```python
from build123d import *

# Parameters (mm, degrees)
SKETCH_1_W          = 25
SKETCH_1_H          = 90
EXTRUDE_1_DEPTH     = 2
SKETCH_3_W          = 2
SKETCH_3_H          = 90
EXTRUDE_2_DEPTH     = 40
SKETCH_6_R          = 1.65
CUT_EXTRUDE_3_DEPTH = 10
SKETCH_7_R          = 3
CUT_EXTRUDE_4_DEPTH = 10
SKETCH_8_R          = 1.65
CUT_EXTRUDE_5_DEPTH = 10
EXTRUDE_3_DEPTH     = 27
SKETCH_10_R         = 1.65
SKETCH_10_R_2       = 2
CUT_EXTRUDE_7_DEPTH = 6


with BuildPart() as part:
    # 草图1 → 凸台-拉伸1 (new body)
    with BuildSketch(Plane(origin=(0, 0, 0), x_dir=(1, 0, 0), z_dir=(0, 1, 0))):
        Rectangle(SKETCH_1_W, SKETCH_1_H)
    extrude(amount=EXTRUDE_1_DEPTH)

    # 草图3 → 凸台-拉伸2 (add)
    with BuildSketch(Plane(origin=(0, 2, 0), x_dir=(1, 0, 0), z_dir=(0, 1, 0))):
        with Locations((-11.5, 0)):
            Rectangle(SKETCH_3_W, SKETCH_3_H)
    extrude(amount=EXTRUDE_2_DEPTH)

    # 草图6 → 切除-拉伸3 (cut)
    with BuildSketch(Plane.ZY.offset(12.5)):
        with Locations((8, 21)):
            Circle(SKETCH_6_R)
        with Locations((21.524795588, 17.383384964)):
            Circle(SKETCH_6_R)
        with Locations((15, 14)):
            Circle(SKETCH_6_R)
        with Locations((15, 28)):
            Circle(SKETCH_6_R)
    extrude(amount=-CUT_EXTRUDE_3_DEPTH, mode=Mode.SUBTRACT)

    # 草图7 → 切除-拉伸4 (cut)
    with BuildSketch(Plane(origin=(0, 0, 0), x_dir=(-1, 0, 0), z_dir=(0, -1, 0))):
        with Locations(Location((-4.5, 28.45, 0), (0, 0, 90))):
            Circle(SKETCH_7_R)
    extrude(amount=-CUT_EXTRUDE_4_DEPTH, mode=Mode.SUBTRACT)

    # 草图8 → 切除-拉伸5 (cut)
    with BuildSketch(Plane(origin=(-10.5, 0, 0), x_dir=(0, 0, -1), z_dir=(1, 0, 0))):
        with Locations((-40, 22)):
            Circle(SKETCH_8_R)
        with Locations((40, 22)):
            Circle(SKETCH_8_R)
    extrude(amount=-CUT_EXTRUDE_5_DEPTH, mode=Mode.SUBTRACT)

    # 草图9 → 凸台-拉伸3 (add)
    with BuildSketch(Plane(origin=(-10.5, 0, 0), x_dir=(0, 0, -1), z_dir=(1, 0, 0))):
        Polygon((-45, 35), (0, 35), (45, 35), (45, 37), (-45, 37), align=None)
    extrude(amount=EXTRUDE_3_DEPTH)

    # 草图10 → 切除-拉伸7 (cut)
    with BuildSketch(Plane.XZ.offset(-35)):
        with Locations(Location((4.5, -17.95, 0), (0, 0, 270))):
            Circle(SKETCH_10_R)
        with Locations(Location((11.5, -10.95, 0), (0, 0, 270))):
            Circle(SKETCH_10_R)
        with Locations(Location((4.5, -10.95, 0), (0, 0, 270))):
            Circle(SKETCH_10_R_2)
        with Locations(Location((-2.5, -10.95, 0), (0, 0, 270))):
            Circle(SKETCH_10_R)
        with Locations(Location((4.5, -3.95, 0), (0, 0, 270))):
            Circle(SKETCH_10_R)
    extrude(amount=-CUT_EXTRUDE_7_DEPTH, mode=Mode.SUBTRACT)


solid = part.part
```
The listing builds one solid part. Answer for the finished solid, in the listing's coordinates (mm). A direction names the side the tool comes from. Give positions to 0.01 mm unless a question says otherwise; leave off trailing zeros. Write each loop counter-clockwise with the first axis right and the second up, starting at its lowest first coordinate (ties: lowest second). Pieces come first, ordered by that corner, then holes. Notation, with made-up numbers: (-20.5, -12.5) -> (15.5, -12.5) arc R38 cw to (15.5, 26.5) -> close; hole circle Ø11 at (63, -10.75). An arc over 180 degrees is marked (long way). Write item = value, one per line. Start each with the question number.
1) Each of these flat-tipped pins is pushed along its axis until it touches: pin 1 (5 mm diameter, centred on x = 4.5, z = -10.95, fed in from +Y); pin 2 (1 mm diameter, centred on y = 1, z = -2, fed in from +X); pin 3 (10 mm diameter, centred on x = -6.5, z = -35, fed in from -Y); pin 4 (10 mm diameter, centred on y = 12.5, z = -6, fed in from +X). Where does it stop, or does it pass through?
2) Straight lines are drawn through the part: line 1 along Y through (x, z) = (1.5, 12); line 2 along Y through (x, z) = (-11.6, -40); line 3 along X through (y, z) = (36.55, -17.95). For each, find the intervals that lie inside material, in ascending order.
3) The part is cut by section A-A, the plane z = -3.95. Determine the outline of the cut face in (x, y), and give its area (3 significant figures).
4) Which of the six approach directions +Z, -Z, +X, -X, +Y, -Y give full straight-line access (tool end or side, diameter ignored) to faces 1 (the face through (12.5, 1, 1)), 2 (the face through (10.868, 35.986, -12.474)), 3 (the face through (4.632, 0.986, -25.453)), 4 (the face through (-10.5, 39, 1))?
5) The part is cut by section C-C, the plane x = 11.5. Determine the outline of the cut face in (y, z).
6) The part is cut by section D-D, the plane y = 9.5. Determine the outline of the cut face in (x, z), and give its area (3 significant figures).
7) The part is cut by section B-B, the plane x = 0. Determine the outline of the cut face in (y, z), and give its area (3 significant figures).
8) Determine the mould class of faces 5 (the face through (0, 0, -1)), 6 (the face through (3.734, 35.986, -12.797)), 7 (the face through (1, 2, -1)), 8 (the face through (-11.51, 29.39, 15.89)) for opening direction Y: +Y half, -Y half, draft (parallel to the pull), parting line (faces both ways), or undercut.
Solutions:
q1.pin_1 = 37
q1.pin_2 = 12.5
q1.pin_3 = 0
q1.pin_4 = -10.5
q2.line_1 = 0 to 2, 35 to 37
q2.line_2 = 0 to 20.35, 23.65 to 42
q2.line_3 = -12.5 to 2.85, 6.15 to 16.5
q3.outline = (-12.5, 0) -> (12.5, 0) -> (12.5, 2) -> (-10.5, 2) -> (-10.5, 35) -> (2.85, 35) -> (2.85, 37) -> (-10.5, 37) -> (-10.5, 42) -> (-12.5, 42) -> close; (6.15, 35) -> (16.5, 35) -> (16.5, 37) -> (6.15, 37) -> close
q3.area = 177 mm²
q4.face_1 = +Z, -Z, +X, -Y
q4.face_2 = +Y
q4.face_3 = -Y
q4.face_4 = +Z, -Z, +X, +Y
q5.outline = (0, -45) -> (2, -45) -> (2, 45) -> (0, 45) -> close; (35, -45) -> (37, -45) -> (37, -12.6) -> (35, -12.6) -> close; (35, -9.3) -> (37, -9.3) -> (37, 45) -> (35, 45) -> close
q6.outline = (-12.5, -45) -> (-10.5, -45) -> (-10.5, 45) -> (-12.5, 45) -> close
q6.area = 180 mm²
q7.outline = (0, -45) -> (2, -45) -> (2, 45) -> (0, 45) -> close; (35, -45) -> (37, -45) -> (37, 45) -> (35, 45) -> close
q7.area = 360 mm²
q8.face_5 = -Y half
q8.face_6 = draft
q8.face_7 = undercut
q8.face_8 = undercut
